The figure shows three views and two pictorial views of one solid part (mm, origin at its lowest corner). Answer the questions. Coordinates: 2 decimals unless noted, no trailing zeros. Order: outer loops, then holes, each group sorted by start corner. A loop starts at its lowest first (then second) coordinate and runs counter-clockwise, first axis right, second up. Notation, with made-up numbers: (60, 7.25) -> (111, 7.25) arc R16 ccw to (111, 20.25) -> close; hole circle Ø8 at (-20.75, -5.75). An arc over 180 degrees is marked (long way). Return JSON: item names as keys, results as strings.
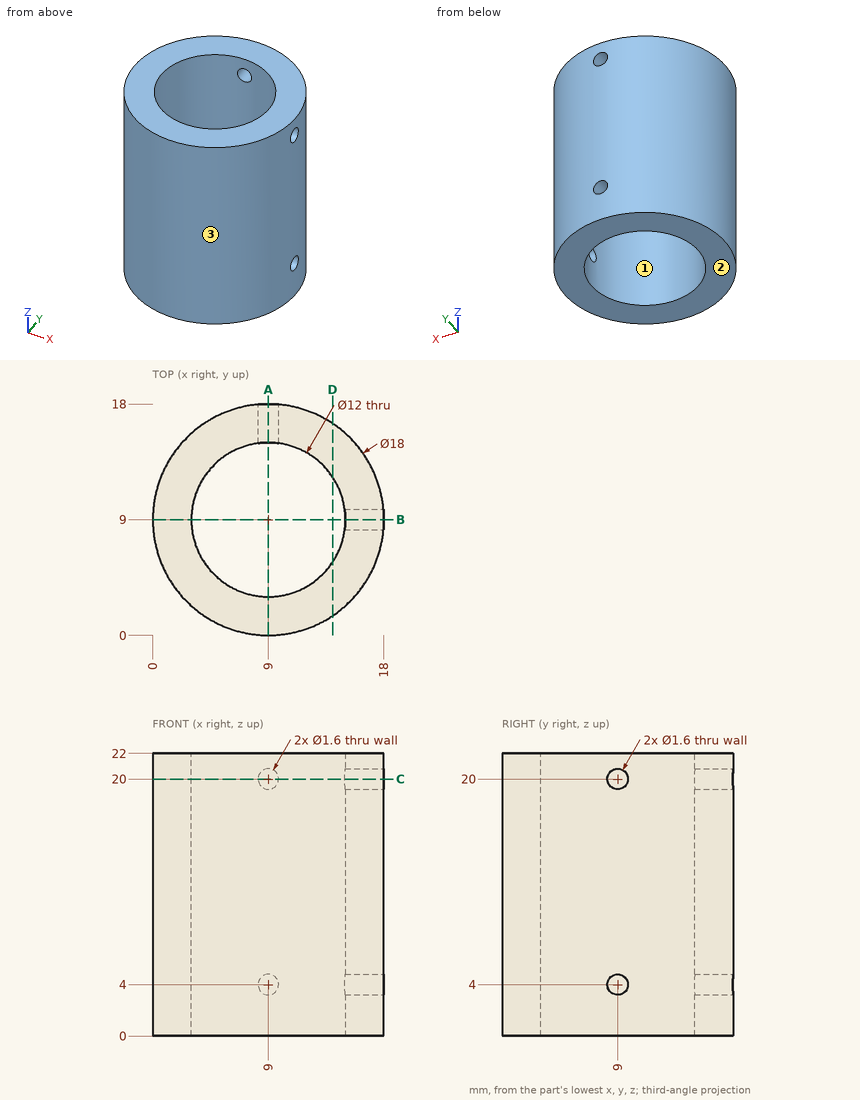
Item 1: Flat-ended cylindrical pins translate along their axes: pin 1 (2 mm diameter, centred on x = 5.5, z = 19.5, fed in from +Y); pin 2 (5 mm diameter, centred on y = 5, z = 4.5, fed in from -X); pin 3 (10 mm diameter, centred on x = 3, z = 6.5, fed in from -Y). Find the tip coordinate at first contact, or state that the pin passes through.
Answer list:
{"pin 1": "y = 17.65", "pin 2": "x = 0.13", "pin 3": "y = 0.06"}
Item 2: The part is cut by section A-A on x = 9. Determine the outline of the cut face in (y, z), plus the area to 3 significant figures.
Answer list:
{"outline": "(0, 0) -> (3, 0) -> (3, 22) -> (0, 22) -> close; (15, 0) -> (18, 0) -> (18, 3.2) -> (15, 3.2) -> close; (15, 4.8) -> (18, 4.8) -> (18, 19.2) -> (15, 19.2) -> close; (15, 20.8) -> (18, 20.8) -> (18, 22) -> (15, 22) -> close", "area": "122 mm2"}
Item 3: The part is cut by section C-C on z = 20. Determine the outline of the cut face in (x, y), plus the area to 3 significant figures.
Answer list:
{"outline": "(8.2, 14.95) -> (8.2, 17.96) arc R9 ccw (long way) to (17.96, 8.2) -> (14.95, 8.2) arc R6 cw (long way) to start; (9.8, 14.95) arc R6 cw to (14.95, 9.8) -> (17.96, 9.8) arc R9 ccw to (9.8, 17.96) -> close", "area": "132 mm2"}
Item 4: Determine the mould class of the marked faces 1, 2 and 3 for opening direction X: pulls with the +X half, pulls with the -X half, needs draft (parallel to the pull), parting line crosses it, or undercut.
Answer list:
{"face 1": "undercut", "face 2": "needs draft", "face 3": "parting line crosses it"}
Item 5: The part is cut by section D-D on x = 14. Determine the outline of the cut face in (y, z), plus the area to 3 significant figures.
Answer list:
{"outline": "(1.52, 0) -> (5.68, 0) -> (5.68, 22) -> (1.52, 22) -> close; (12.32, 0) -> (16.48, 0) -> (16.48, 22) -> (12.32, 22) -> close", "area": "183 mm2"}
Item 6: Find the intervals of material crossed by probe 1 along Y at (x, z) = (9, 6.75); probe 2 along X at (y, z) = (10.5, 11.25); probe 3 along Y at (x, z) = (4, 5), in increasing order.
Answer list:
{"probe 1": "0 to 3, 15 to 18", "probe 2": "0.13 to 3.19, 14.81 to 17.87", "probe 3": "1.52 to 5.68, 12.32 to 16.48"}
